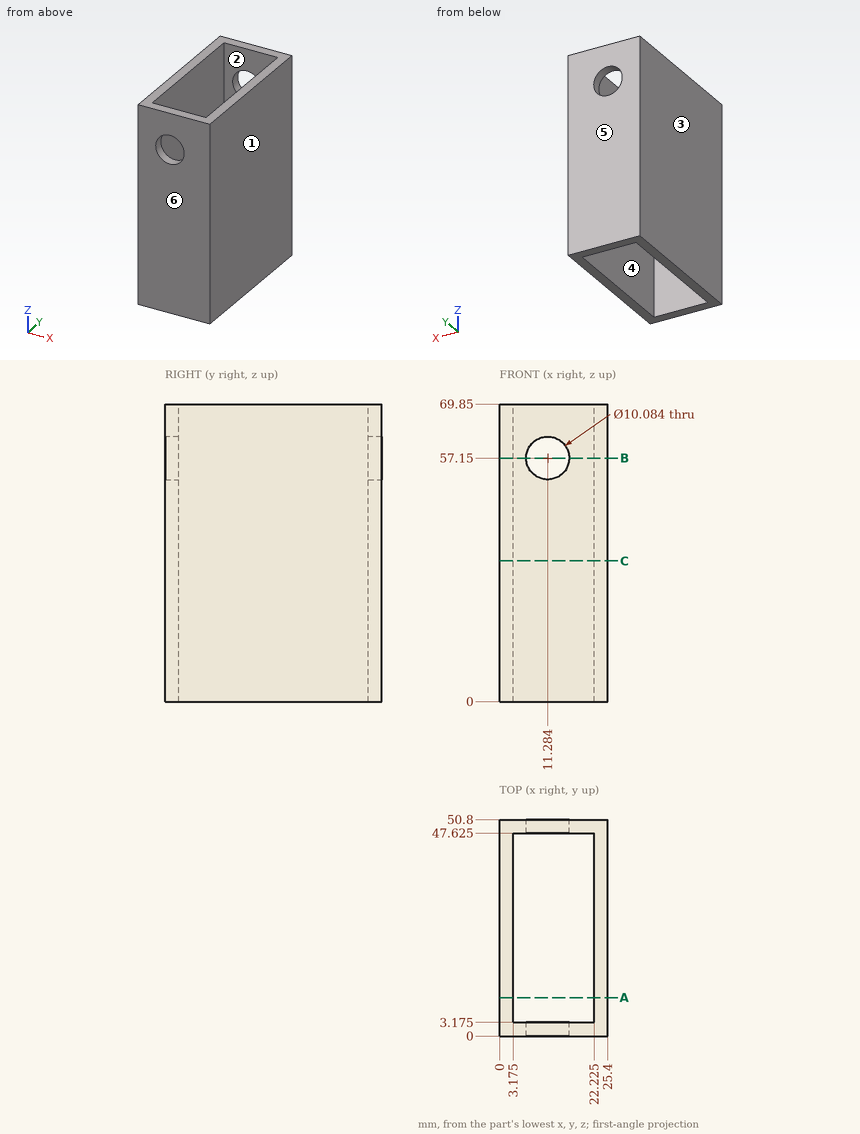
Study the drawing (mm; zero at the part's minimum x, y, z) and answer. A direction names the side the tool comes from. Coordinates: 2 decimals unless noted, no trailing zeros. Order: outer loops, then holes, each group sorted by start corner. A loop starts at its lowest first (then second) coordinate and runs counter-clockwise, first axis right, second up. Notation, with made-up numbers: (33.5, -35) -> (49.5, -35) arc R18 ccw to (49.5, -18) -> close; hole circle Ø9 at (34, 75). An arc over 180 degrees is marked (long way). Answer in a Markdown table with one row per item. Add a question column.
Item 1: Find section C-C (z = 33). Write down the section's boundary in (x, y) (3 decimals).
Item 2: Which of the six approach directions +Z, -Z, +X, -X, +Y, -Y give full straight-line access (tool end or side, diameter ignored) to the marked faces 1 and 2?
Item 3: Find the intervals of material crossed by L1, parallel to X at y = 2.35, z = 57.15; L2, parallel to X at y = 6, z = 11.5 (3 decimals); L3, parallel to Y at x = 11.25, z = 14 (3 decimals), in increasing order. Write a range as from..to.
Item 4: This flat-tipped pin is pushed along its axis until it touches: P1, Ø2, axis at x = 7.5, z = 59.5, coming from the +Y side. Where does it stop, or does it pass through?
Item 5: Determine the mould class of the marked faces 3, 4, 5 and 6 for opening direction Y: +Y half, -Y half, draft (parallel to the pull), parting line (faces both ways), or undercut.
Item 6: Find section B-B (z = 57.15). Write down the section's boundary in (x, y) (1 decimal).
Item 7: Find section A-A (y = 9). Write down the section's boundary in (x, z) (3 decimals).
Result set:
| question | item | result |
|---|---|---|
| 1 | outline | (0, 0) -> (25.4, 0) -> (25.4, 50.8) -> (0, 50.8) -> close; hole (3.175, 3.175) -> (22.225, 3.175) -> (22.225, 47.625) -> (3.175, 47.625) -> close |
| 2 | face 1 | +Z, -Z, +X, +Y, -Y |
| 2 | face 2 | +Z, -Z |
| 3 | L1 | x = 0..6.24, 16.33..25.4 |
| 3 | L2 | x = 0..3.175, 22.225..25.4 |
| 3 | L3 | y = 0..3.175, 47.625..50.8 |
| 4 | P1 | stops at y = 50.8 |
| 5 | face 3 | draft |
| 5 | face 4 | undercut |
| 5 | face 5 | +Y half |
| 5 | face 6 | -Y half |
| 6 | outline | (0, 0) -> (6.2, 0) -> (6.2, 3.2) -> (3.2, 3.2) -> (3.2, 47.6) -> (6.2, 47.6) -> (6.2, 50.8) -> (0, 50.8) -> close; (16.3, 0) -> (25.4, 0) -> (25.4, 50.8) -> (16.3, 50.8) -> (16.3, 47.6) -> (22.2, 47.6) -> (22.2, 3.2) -> (16.3, 3.2) -> close |
| 7 | outline | (0, 0) -> (3.175, 0) -> (3.175, 69.85) -> (0, 69.85) -> close; (22.225, 0) -> (25.4, 0) -> (25.4, 69.85) -> (22.225, 69.85) -> close |
